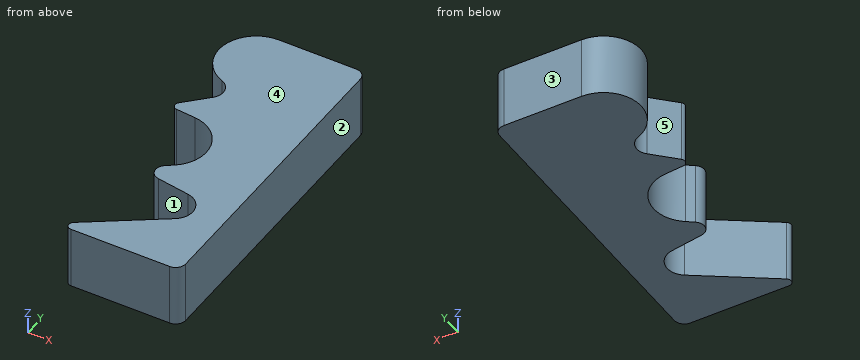
from build123d import *

# Parameters (mm, degrees)
F1_DEPTH = 1.5875


with BuildPart() as f1:
    # F0 (on Top) → F1 (new body, symmetric)
    with BuildSketch(Plane.XY):
        with BuildLine():
            Line((-5.524762, 0), (-0.508, 0))
            ThreePointArc((-0.508, 0), (-0.14879, 0.14879), (0, 0.508))
            Line((0, 0.508), (0, 15.367))
            ThreePointArc((0, 15.367), (-0.14879, 15.72621), (-0.508, 15.875))
            Line((-0.508, 15.875), (-4.445, 15.875))
            ThreePointArc((-4.445, 15.875), (-6.318154, 14.316871), (-5.127144, 12.191319))
            ThreePointArc((-5.127144, 12.191319), (-4.677356, 11.664932), (-4.873952, 11.001048))
            Line((-4.873952, 11.001048), (-5.964836, 9.910164))
            ThreePointArc((-5.964836, 9.910164), (-6.023912, 9.643686), (-5.807368, 9.477526))
            Line((-5.807368, 9.477526), (-4.828483, 9.391884))
            ThreePointArc((-4.828483, 9.391884), (-3.240143, 8.070876), (-3.921246, 6.120495))
            Line((-3.921246, 6.120495), (-4.264111, 5.871389))
            ThreePointArc((-4.264111, 5.871389), (-4.45948, 5.341818), (-4.044985, 4.958663))
            Line((-4.044985, 4.958663), (-2.379395, 4.694859))
            ThreePointArc((-2.379395, 4.694859), (-1.597478, 3.960691), (-1.992111, 2.963365))
            Line((-1.992111, 2.963365), (-5.667589, 0.464039))
            ThreePointArc((-5.667589, 0.464039), (-5.767524, 0.17928), (-5.524762, 0))
        make_face()
    extrude(amount=F1_DEPTH, both=True)


solid = f1.part
Geometry check sheet. Reference: the model listing, model coordinates, mm. Face numbers are marked on the shaded views. A direction names the side the tool comes from. Round coordinates to 2 decimals unless told otherwise and drop trailing zeros. Write each loop counter-clockwise with the first axis right and the second up, starting at its lowest first coordinate (ties: lowest second). Pieces come first, ordered by that corner, then holes. Notation, with made-up numbers: (32, 16.25) -> (57, 16.25) arc R17 ccw to (57, 25.25) -> close; hole circle Ø10 at (63, 89.5). An arc over 180 degrees is marked (long way). One line per item, written item: value. Start each with the question number.
(1) Draft check along Y on the marked faces 3, 4 and 5. Enter one of: +Y half, -Y half, draft (parallel to the pull), parting line (faces both ways), or undercut.
(2) Scan lines: line 1 (Y direction, x = -4, z = -0.75) (3 decimals); line 2 (Y direction, x = -3.75, z = -0.75) (3 decimals); line 3 (Y direction, x = -2, z = 0.2) (3 decimals). Record each from-to range of solid material in increasing order. Write a range as [from, to].
(3) Access from +Z, -Z, +X, -X, +Y, -Y to the whole of each face (thin tool, end or side, straight path). Record for the marked faces 1 and 2.
(4) Cross-section at A-A, the plane x = -2.75. Record the cut outline in (y, z) (1 decimal), and give its area (3 significant figures).
(5) Cross-section at B-B, the plane z = -0.05. Record the cut outline in (x, y) (1 decimal), and give its area (3 significant figures).
(6) Cross-section at C-C, the plane y = 14.75. Record the cut outline in (x, z), and give its area (3 significant figures).
(7) Cross-section at D-D, the plane y = 12.5. Record the cut outline in (x, z).
(8) Go/stop test with a flat-tipped pin: pin 1 Ø1.5 at (y, z) = (9, 1) entering from -X. Record where the tip stops, or that it passes through.
Answer:
1. face 3: +Y half
1. face 4: draft
1. face 5: undercut
2. line 1: [0, 1.598], [4.952, 6.063], [9.107, 15.875]
2. line 2: [0, 1.768], [4.912, 6.262], [8.911, 15.875]
2. line 3: [0, 2.958], [4.547, 15.875]
3. face 1: +Z, -Z, -X
3. face 2: +Z, -Z, +X, +Y, -Y
4. outline: (0, -1.6) -> (2.4, -1.6) -> (2.4, 1.6) -> (0, 1.6) -> close; (4.8, -1.6) -> (15.9, -1.6) -> (15.9, 1.6) -> (4.8, 1.6) -> close
4. area: 43.1 mm²
5. outline: (-6, 9.9) arc R0.3 ccw to (-5.8, 9.5) -> (-4.8, 9.4) arc R1.8 cw to (-3.9, 6.1) -> (-4.3, 5.9) arc R0.5 ccw to (-4, 5) -> (-2.4, 4.7) arc R1 cw to (-2, 3) -> (-5.7, 0.5) arc R0.3 ccw to (-5.5, 0) -> (-0.5, 0) arc R0.5 ccw to (0, 0.5) -> (0, 15.4) arc R0.5 ccw to (-0.5, 15.9) -> (-4.4, 15.9) arc R1.9 ccw to (-5.1, 12.2) arc R0.7 cw to (-4.9, 11) -> close
5. area: 69.1 mm²
6. outline: (-6.18, -1.59) -> (0, -1.59) -> (0, 1.59) -> (-6.18, 1.59) -> close
6. area: 19.6 mm²
7. outline: (-5.66, -1.59) -> (0, -1.59) -> (0, 1.59) -> (-5.66, 1.59) -> close
8. pin 1: x = -6.04
